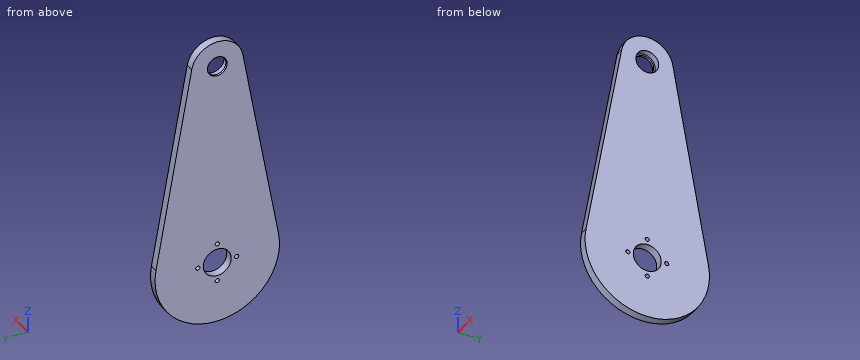
from build123d import *

# Parameters (mm, degrees)
SKETCH1_R           = 13.5
SKETCH1_R_2         = 11
BOSS_EXTRUDE1_DEPTH = 4
SKETCH2_R           = 2
CUT_EXTRUDE1_DEPTH  = 234
SKETCH3_R           = 11
SKETCH3_R_2         = 9.5
BOSS_EXTRUDE3_DEPTH = 2


with BuildPart() as part:
    # Sketch1 → Boss-Extrude1 (new, symmetric)
    with BuildSketch(Plane(origin=(0, 0, 0), x_dir=(0, 0, -1), z_dir=(1, 0, 0))):
        with BuildLine():
            Line((-204.375, 24.614210834), (-10.5, 59.074106003))
            ThreePointArc((-10.5, 59.074106003), (60, 0), (-10.5, -59.074106003))
            Line((-10.5, -59.074106003), (-204.375, -24.614210834))
            ThreePointArc((-204.375, -24.614210834), (-225, 0), (-204.375, 24.614210834))
        make_face()
        Circle(SKETCH1_R, mode=Mode.SUBTRACT)
        with Locations((-200, 0)):
            Circle(SKETCH1_R_2, mode=Mode.SUBTRACT)
    extrude(amount=BOSS_EXTRUDE1_DEPTH, both=True)

    # Sketch2 → Cut-Extrude1 (cut, through all)
    with BuildSketch(Plane(origin=(4, 0, 0), x_dir=(0, 0, -1), z_dir=(1, 0, 0))):
        with Locations((0, 18.75)):
            Circle(SKETCH2_R)
        with Locations((18.75, 0)):
            Circle(SKETCH2_R)
        with Locations((0, -18.75)):
            Circle(SKETCH2_R)
        with Locations((-18.75, 0)):
            Circle(SKETCH2_R)
    extrude(amount=-CUT_EXTRUDE1_DEPTH, mode=Mode.SUBTRACT)

    # Sketch3 → Boss-Extrude3 (add)
    with BuildSketch(Plane.ZY.offset(4)):
        with Locations((200, 0)):
            Circle(SKETCH3_R)
        with Locations((200, 0)):
            Circle(SKETCH3_R_2, mode=Mode.SUBTRACT)
    extrude(amount=-BOSS_EXTRUDE3_DEPTH)


solid = part.part
The model under review builds one solid part; all positions refer to its coordinate system, in mm. Round coordinates to 2 decimals unless told otherwise and drop trailing zeros. Write each loop counter-clockwise with the first axis right and the second up, starting at its lowest first coordinate (ties: lowest second). Pieces come first, ordered by that corner, then holes. Notation, with made-up numbers: M 16.25,-38.75 L 35.25,-38.75 A23 ccw 35.25,-22.75 Z; hole C -37.75,39 d1. An arc over 180 degrees is marked long. Use a Markdown table: item, result. Add a question column.
Q1. To check wall thickness, follow line 1 (Y direction, x = 1.75, z = 0); line 2 (Y direction, x = -2.55, z = 200); line 3 (Y direction, x = 0, z = 195). State the ranges of each line that lie inside material, in increasing order.
Q2. We need section D-D, the plane z = 36.5. State the section outline as (x, y) points.
Q3. We need section B-B, the plane y = 6. State the section outline as (x, z) points.
Q4. We need section C-C, the plane z = 197. State the section outline as (x, y) points.
Q5. We need section A-A, the plane x = 0.5. State the section outline as (y, z) points (3 decimals), plus the area to 3 significant figures.
Q6. Insertion check: pin 1 (24.5 mm diameter, centred on y = 0, z = 0, fed in from -X); pin 2 (1 mm diameter, centred on x = -0.5, z = -12.5, fed in from +Y); pin 3 (2 mm diameter, centred on x = 1, z = 49.5, fed in from -Y); pin 4 (3 mm diameter, centred on x = 2.5, y = 2, fed in from -Z). Each pin has a flat end and moves straight along its axis. Give the tip position at first contact, or say it passes through.
Findings below:
| question | item | result |
|---|---|---|
| 1 | line 1 | y = -60 to -20.75, -16.75 to -13.5, 13.5 to 16.75, 20.75 to 60 |
| 1 | line 2 | y = -25.39 to -9.5, 9.5 to 25.39 |
| 1 | line 3 | y = -26.28 to -9.8, 9.8 to 26.28 |
| 2 | outline | M -4,-54.45 L 4,-54.45 L 4,54.45 L -4,54.45 Z |
| 3 | outline | M -4,-59.7 L 4,-59.7 L 4,-12.09 L -4,-12.09 Z; M -4,12.09 L 4,12.09 L 4,190.78 L -2,190.78 L -2,192.63 L -4,192.63 Z; M -4,207.37 L -2,207.37 L -2,209.22 L 4,209.22 L 4,224.27 L -4,224.27 Z |
| 4 | outline | M -4,-25.93 L 4,-25.93 L 4,-10.58 L -2,-10.58 L -2,-9.01 L -4,-9.01 Z; M -4,9.01 L -2,9.01 L -2,10.58 L 4,10.58 L 4,25.93 L -4,25.93 Z |
| 5 | outline | M -59.074,10.5 A60 ccw long 59.074,10.5 L 24.614,204.375 A25 ccw -24.614,204.375 Z; hole C -18.75,0 d4; hole C 0,0 d27; hole C 0,200 d22; hole C 0,-18.75 d4; hole C 0,18.75 d4; hole C 18.75,0 d4 |
| 5 | area | 22,900 mm² |
| 6 | pin 1 | passes through |
| 6 | pin 2 | stops at y = 58.79 |
| 6 | pin 3 | stops at y = -52.32 |
| 6 | pin 4 | stops at z = -60 |
